Autodesk Inventor part; units mm, degrees
ref_plane "YZ Plane" through (0, 0, 0) normal (1, 0, 0) x (0, 1, 0)
ref_plane "XZ Plane" through (0, 0, 0) normal (0, 1, 0) x (-1, 0, 0)
ref_plane "XY Plane" through (0, 0, 0) normal (0, 0, 1) x (1, 0, 0)
sketch "Sketch1" plane through (0, 0, 0) normal (0, 0, 1) x (1, 0, 0)
  line L0 (-6.25, -7.25) -> (6.25, -7.25)
  line L1 (6.25, -7.25) -> (6.25, 7.25)
  line L2 (6.25, 7.25) -> (-6.25, 7.25)
  line L3 (-6.25, 7.25) -> (-6.25, -7.25)
  line L4 (-6.25, -7.25) -> (6.25, 7.25) construction
  line L5 (6.25, -7.25) -> (-6.25, 7.25) construction
  line L6 (-8.75, -9.75) -> (8.75, -9.75)
  line L7 (8.75, -9.75) -> (8.75, 9.75)
  line L8 (8.75, 9.75) -> (-8.75, 9.75)
  line L9 (-8.75, 9.75) -> (-8.75, -9.75)
  line L10 (-8.75, -9.75) -> (8.75, 9.75) construction
  line L11 (8.75, -9.75) -> (-8.75, 9.75) construction
  line L12 (-3.75, -4.75) -> (3.75, -4.75)
  line L13 (3.75, -4.75) -> (3.75, 4.75)
  line L14 (3.75, 4.75) -> (-3.75, 4.75)
  line L15 (-3.75, 4.75) -> (-3.75, -4.75)
  line L16 (-3.75, -4.75) -> (3.75, 4.75) construction
  line L17 (3.75, -4.75) -> (-3.75, 4.75) construction
  point P0 (0, 0)
  dimension "d0" = 12.5
  dimension "d1" = 14.5
  dimension "d2" = 17.5
  dimension "d3" = 19.5
  dimension "d4" = 7.5
  dimension "d5" = 9.5
extrude "Extrusion1" add sketch "Sketch1" along normal blind 2.5 contours L3 L2 L1 L0 | L9 L8 L7 L6
extrude "Extrusion2" add sketch "Sketch1" against normal blind 7.5 contours L9 L8 L7 L6
sketch "Sketch2" plane through (0, 0, 2.5) normal (0, 0, 1) x (1, 0, 0)
  line L0 (-8.75, -9.75) -> (-8.75, 9.75)
  line L1 (-3.75, -4.75) -> (-8.75, -4.75)
  line L2 (-8.75, -4.75) -> (-8.75, 4.75)
  line L3 (-8.75, 4.75) -> (-3.75, 4.75)
  line L4 (-3.75, 4.75) -> (-3.75, -4.75)
  line L5 (-3.75, -4.75) -> (-3.75, 4.75)
  point P0 (0, 0)
  point P1 (-3.75, 0)
extrude "Extrusion3" cut sketch "Sketch2" against normal through all
thicken "Thicken1" operation add thickness 10.199 both sides no extend neighbours no toward (0, 1, 0) faces at (2.9167, 9.75, -0.8333)
sketch "Sketch3" plane through (-8.75, 19.949, 2.5) normal (0, 1, 0) x (1, 0, 0)
  line L0 (0, 10) -> (0, 0)
  point P0 (8.75, 2.5)
  point P1 (5, 5)
  point P2 (0, 5)
  dimension "d22" = 5
hole "Hole1" at (-3.75, 19.949, -2.5) direction (0, -1, 0) diameter 5.35 depth 10 tip angle 118
properties part number "Adafruit_1528_4663-ND_House_01"
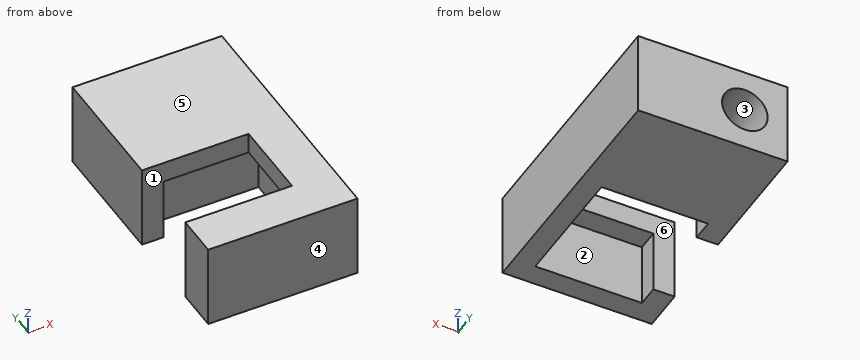
The model under review builds one solid part; all positions refer to its coordinate system, in mm. Face numbers are marked on the shaded views. A direction names the side the tool comes from. Give positions to 0.01 mm unless a question says otherwise; leave off trailing zeros. Loops run counter-clockwise (first coordinate to the right, second up) from the corner with the lowest first, then second, coordinate; pieces in that order, holes last. Notation, with made-up numbers: (48, -2.75) -> (52, -2.75) arc R21 cw to (52, 14.25) -> close; hole circle Ø2 at (71, 19). An arc over 180 degrees is marked (long way). Put each result on its own line as item: value. Start each with the question number.
1. For the marked faces 1, 2 and 3, list the 3-axis set-ups (+Z, -Z, +X, -X, +Y, -Y) from which the entire face can be reached by the end or side of a thin tool; tool diameter is ignored.
2. We need section D-D on x = 4.75. State the section outline as (y, z) points.
3. Wall thickness on probe 1 along Y at (x, z) = (-7.5, 2); probe 2 along X at (y, z) = (14.5, -2.5) (3 decimals); probe 3 along Z at (x, y) = (-3.75, 17.5) (3 decimals): over which ranges is each line inside the solid? List them lowest first.
4. We need section C-C on x = 1.25. State the section outline as (y, z) points.
5. Mouldability with a two-part tool opening along Y and no side actions: class the marked faces 4, 5 and 6 as released by +Y, released by -Y, zero draft, split by the parting line, or undercut.
6. Clearance check with flat-ended pins moving along their axes: P1, Ø4, axis at x = 1.5, y = 2.5, coming from the -Z side; P2, Ø3, axis at y = -0.5, z = 0.5, coming from the -X side; P3, Ø5, axis at x = -3.75, z = -2.5, coming from the +Y side; P4, Ø2, axis at y = 0, z = -3, coming from the -X side. State where each tip first meets the part, or that it passes through.
7. We need section B-B on z = -6. State the section outline as (x, y) points.
8. We need section A-A on y = 13. State the section outline as (x, z) points (3 decimals), then the cut area to 3 significant figures.
Determined:
1. face 1: +Z, -Z, -X
1. face 2: -Z
1. face 3: +Y
2. outline: (-9.75, -7.5) -> (-7.25, -7.5) -> (-7.25, 0) -> (7.25, 0) -> (7.25, -7.5) -> (19.95, -7.5) -> (19.95, 2.5) -> (-9.75, 2.5) -> close
3. probe 1: -9.75 to -4.75, 4.75 to 19.95
3. probe 2: -8.75 to -6.425, -1.075 to 8.75
3. probe 3: -7.5 to -5.175, 0.175 to 2.5
4. outline: (-9.75, -7.5) -> (-7.25, -7.5) -> (-7.25, 0) -> (-4.75, 0) -> (-4.75, 2.5) -> (-9.75, 2.5) -> close; (4.75, 0) -> (7.25, 0) -> (7.25, -7.5) -> (19.95, -7.5) -> (19.95, 2.5) -> (4.75, 2.5) -> close
5. face 4: released by -Y
5. face 5: zero draft
5. face 6: undercut
6. P1: through
6. P2: x = 3.75
6. P3: y = 9.84
6. P4: x = 6.25
7. outline: (-8.75, -9.75) -> (8.75, -9.75) -> (8.75, 19.95) -> (-8.75, 19.95) -> (-8.75, 4.75) -> (-6.25, 4.75) -> (-6.25, 7.25) -> (6.25, 7.25) -> (6.25, -7.25) -> (-6.25, -7.25) -> (-6.25, -4.75) -> (-8.75, -4.75) -> close
8. outline: (-8.75, -7.5) -> (8.75, -7.5) -> (8.75, 2.5) -> (-8.75, 2.5) -> close; hole circle Ø5.35 at (-3.75, -2.5)
8. area: 153 mm^2
